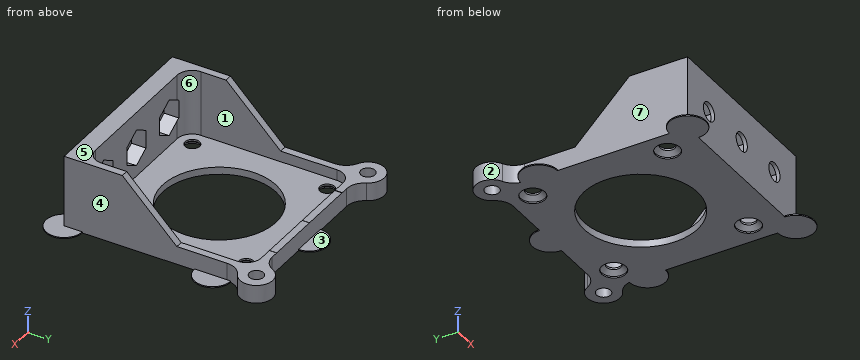
from build123d import *
from build123d.topology import SkipClean

# Parameters (mm, degrees)
SKETCH3_R                                     = 19.812
SKETCH3_R_2                                   = 2.55
BOSS_EXTRUDE1_DEPTH                           = 2.54
BOSS_EXTRUDE6_DEPTH                           = 3.81
BOSS_EXTRUDE10_DEPTH                          = 22.86
BOSS_EXTRUDE10_DEPTH_BACK                     = 2.54
CHAMFER1_SIZE                                 = 20.32
CUT_EXTRUDE2_DEPTH                            = 5.08
CUT_EXTRUDE2_DEPTH_BACK                       = 73.755970889
F_1_4_CLEARANCE_HOLE1_D                       = 6.5278
SKETCH22_R                                    = 2.413
BOSS_EXTRUDE18_DEPTH                          = 6.35
FILLET1_R                                     = 6.35
CSK_FOR_FLAT_HEAD_MACHINE_SCREW_100_1_A_COUNT = 2
CSK_FOR_FLAT_HEAD_MACHINE_SCREW_100_1_A_PITCH = 47.14
CSK_FOR_FLAT_HEAD_MACHINE_SCREW_100_2_COUNT   = 2
CSK_FOR_FLAT_HEAD_MACHINE_SCREW_100_2_PITCH   = 66.66602733
CSK_FOR_FLAT_HEAD_MACHINE_SCREW_100_3_COUNT   = 2
CSK_FOR_FLAT_HEAD_MACHINE_SCREW_100_3_PITCH   = 47.14
F_10_CLEARANCE_HOLE1_D                        = 4.9784
SKETCH6_R                                     = 6.35
TABS_DEPTH                                    = 0.4


with BuildPart() as part:
    # Sketch3 → Boss-Extrude1 (new body)
    with BuildSketch(Plane.XY):
        with BuildLine():
            Line((23.755, 31.502), (-23.755, 31.502))
            ThreePointArc((-23.755, 31.502), (-29.232956234, 29.232956234), (-31.502, 23.755))
            Line((-31.502, 23.755), (-31.502, -23.755))
            ThreePointArc((-31.502, -23.755), (-29.232956234, -29.232956234), (-23.755, -31.502))
            Line((-23.755, -31.502), (23.755, -31.502))
            ThreePointArc((23.755, -31.502), (29.232956234, -29.232956234), (31.502, -23.755))
            Line((31.502, -23.755), (31.502, 23.755))
            ThreePointArc((31.502, 23.755), (29.232956234, 29.232956234), (23.755, 31.502))
        make_face()
        Circle(SKETCH3_R, mode=Mode.SUBTRACT)
        with Locations((23.57, 23.57)):
            Circle(SKETCH3_R_2, mode=Mode.SUBTRACT)
        with Locations((-23.57, 23.57)):
            Circle(SKETCH3_R_2, mode=Mode.SUBTRACT)
        with Locations((-23.57, -23.57)):
            Circle(SKETCH3_R_2, mode=Mode.SUBTRACT)
        with Locations((23.57, -23.57)):
            Circle(SKETCH3_R_2, mode=Mode.SUBTRACT)
    extrude(amount=BOSS_EXTRUDE1_DEPTH)

    # Sketch16 → Boss-Extrude6 (add)
    with BuildSketch(Plane.XY.offset(2.54)):
        with BuildLine():
            Line((23.755, 31.502), (-23.755, 31.502))
            ThreePointArc((-23.755, 31.502), (-29.232956234, 29.232956234), (-31.502, 23.755))
            Line((-31.502, 23.755), (-31.502, -23.755))
            ThreePointArc((-31.502, -23.755), (-29.232956234, -29.232956234), (-23.755, -31.502))
            Line((-23.755, -31.502), (23.755, -31.502))
            ThreePointArc((23.755, -31.502), (29.232956234, -29.232956234), (31.502, -23.755))
            Line((31.502, -23.755), (31.502, 23.755))
            ThreePointArc((31.502, 23.755), (29.232956234, 29.232956234), (23.755, 31.502))
        make_face()
        with BuildLine():
            Line((23.755, 28.962), (-23.755, 28.962))
            ThreePointArc((-23.755, 28.962), (-27.43690501, 27.43690501), (-28.962, 23.755))
            Line((-28.962, 23.755), (-28.962, -23.755))
            ThreePointArc((-28.962, -23.755), (-27.43690501, -27.43690501), (-23.755, -28.962))
            Line((-23.755, -28.962), (23.755, -28.962))
            ThreePointArc((23.755, -28.962), (27.43690501, -27.43690501), (28.962, -23.755))
            Line((28.962, -23.755), (28.962, 23.755))
            ThreePointArc((28.962, 23.755), (27.43690501, 27.43690501), (23.755, 28.962))
        make_face(mode=Mode.SUBTRACT)
    extrude(amount=BOSS_EXTRUDE6_DEPTH)

    # Sketch17 → Boss-Extrude10 (add, two sides: drawn at the far end of the back side and taken through both)
    with SkipClean():  # the faces are left unmerged after this step: merging them gives an invalid solid
        with BuildSketch(Plane.XY.offset(2.54).offset(-BOSS_EXTRUDE10_DEPTH_BACK)):
            with BuildLine():
                Line((-31.502, -35.312), (31.502, -35.312))
                Line((31.502, -35.312), (31.502, -16.262))
                Line((31.502, -16.262), (28.962, -16.262))
                Line((28.962, -16.262), (28.962, -23.755))
                ThreePointArc((28.962, -23.755), (27.43690501, -27.43690501), (23.755, -28.962))
                Line((23.755, -28.962), (-23.755, -28.962))
                ThreePointArc((-23.755, -28.962), (-27.43690501, -27.43690501), (-28.962, -23.755))
                Line((-28.962, -23.755), (-28.962, -16.262))
                Line((-28.962, -16.262), (-31.502, -16.262))
                Line((-31.502, -16.262), (-31.502, -35.312))
            make_face()
        extrude(amount=BOSS_EXTRUDE10_DEPTH + BOSS_EXTRUDE10_DEPTH_BACK)
    add(part.part.scale(1), mode=Mode.REPLACE)  # the faces are merged on a copy

    # Chamfer1
    # the kernel refuses this chamfer: 20.32 mm, written as the material it adds along each edge
    with BuildSketch(Plane(origin=(28.962, -16.262, 6.35), x_dir=(0, -0.02749587661058643, 0.9996219169112968), z_dir=(1, 0, 0))) as chamfer1_piece_1_section:
        Polygon((CHAMFER1_SIZE * 0.999621916911, -CHAMFER1_SIZE * 0.0274958766106), (-CHAMFER1_SIZE * 0.0274958766106, -CHAMFER1_SIZE * 0.999621916911), (0, 0), align=None)
    chamfer1_piece_1 = extrude(amount=2.54, mode=Mode.PRIVATE)
    chamfer1_piece_1 = split(chamfer1_piece_1, bisect_by=Plane(origin=(30.232, -9.48984053, 25.4), z_dir=(0, 0, -1)), keep=Keep.TOP, mode=Mode.PRIVATE)
    add(chamfer1_piece_1)
    with BuildSketch(Plane(origin=(-31.502, -16.262, 6.35), x_dir=(0, -0.02749587661058643, 0.9996219169112968), z_dir=(1, 0, 0))) as chamfer1_piece_2_section:
        Polygon((CHAMFER1_SIZE * 0.999621916911, -CHAMFER1_SIZE * 0.0274958766106), (-CHAMFER1_SIZE * 0.0274958766106, -CHAMFER1_SIZE * 0.999621916911), (0, 0), align=None)
    chamfer1_piece_2 = extrude(amount=2.54, mode=Mode.PRIVATE)
    chamfer1_piece_2 = split(chamfer1_piece_2, bisect_by=Plane(origin=(-30.232, -9.48984053, 25.4), z_dir=(0, 0, -1)), keep=Keep.TOP, mode=Mode.PRIVATE)
    add(chamfer1_piece_2)

    # Sketch18 → Cut-Extrude2 (cut, two sides: drawn at the far end of the back side and taken through both)
    with BuildSketch(Plane.XZ.offset(28.962).offset(-CUT_EXTRUDE2_DEPTH_BACK)):
        Polygon((0, 19.079143124), (-5.5245, 15.889571562), (-5.5245, 9.510428438), (0, 6.320856876), (5.5245, 9.510428438), (5.5245, 15.889571562), align=None)
        Polygon((-24.5745, 15.889571562), (-19.05, 19.079143124), (-13.5255, 15.889571562), (-13.5255, 9.510428438), (-19.05, 6.320856876), (-24.5745, 9.510428438), align=None)
        Polygon((19.05, 19.079143124), (13.5255, 15.889571562), (13.5255, 9.510428438), (19.05, 6.320856876), (24.5745, 9.510428438), (24.5745, 15.889571562), align=None)
    extrude(amount=CUT_EXTRUDE2_DEPTH + CUT_EXTRUDE2_DEPTH_BACK, mode=Mode.SUBTRACT)

    # 1/4 Clearance Hole1 (through all)
    with Locations(Plane(origin=(0, -34.042, 0), x_dir=(1, 0, 0), z_dir=(0, 1, 0))):
        with Locations((-19.05, -12.7), (0, -12.7), (19.05, -12.7)):
            Hole(F_1_4_CLEARANCE_HOLE1_D / 2)

    # Sketch22 → Boss-Extrude18 (add)
    with BuildSketch(Plane(origin=(0, 0, 0), x_dir=(-1, 0, 0), z_dir=(0, 0, -1))):
        with BuildLine():
            ThreePointArc((-27.002557269, 30.78844729), (-26.814125955, 31.617757649), (-26.750848437, 32.465848437))
            ThreePointArc((-26.750848437, 32.465848437), (-37.061910478, 35.862528982), (-30.78844729, 27.002557269))
            ThreePointArc((-30.78844729, 27.002557269), (-29.232956234, 29.232956234), (-27.002557269, 30.78844729))
        make_face()
        with Locations((-32.465848437, 32.465848437)):
            Circle(SKETCH22_R, mode=Mode.SUBTRACT)
    boss_extrude18 = extrude(amount=-BOSS_EXTRUDE18_DEPTH)

    # Mirror3: Boss-Extrude18 across plane
    add(boss_extrude18.mirror(Plane(origin=(0, 0, 0), x_dir=(0, 0, 1), z_dir=(1, 0, 0))))

    # Fillet1
    fillet1_edges = [part.edges().sort_by_distance(p)[0] for p in [
        (27.002557269, 30.78844729, 3.175),
        (30.78844729, 27.002557269, 3.175),
        (-27.002557269, 30.78844729, 3.175),
        (-30.78844729, 27.002557269, 3.175),
    ]]
    fillet(fillet1_edges, radius=FILLET1_R)

    # Sketch23 → CSK for  Flat Head Machine Screw (100)1 (revolve, cut)
    with BuildSketch(Plane(origin=(23.57, 23.57, 0), x_dir=(0, 1, 0), z_dir=(1, 0, 0))):
        Polygon((0, 0), (0, 25.4), (2.4892, 25.4), (2.4892, 1.957292137), (4.216399111, 0.508), (4.216399111, 0), align=None)
    csk_for_flat_head_machine_screw_100_1 = revolve(axis=Axis((23.57, 23.57, -6.35), (0, 0, 1)), mode=Mode.SUBTRACT)

    # CSK for  Flat Head Machine Screw (100)1 a: CSK for  Flat Head Machine Screw (100)1 ×2
    with Locations(*[(-i * CSK_FOR_FLAT_HEAD_MACHINE_SCREW_100_1_A_PITCH, 0, 0) for i in range(1, CSK_FOR_FLAT_HEAD_MACHINE_SCREW_100_1_A_COUNT)]):
        add(csk_for_flat_head_machine_screw_100_1, mode=Mode.SUBTRACT)

    # CSK for Flat Head Machine Screw _100 2: CSK for  Flat Head Machine Screw (100)1 ×2
    with Locations(*[Vector(-0.7071067811865476, -0.7071067811865476, 0) * (i * CSK_FOR_FLAT_HEAD_MACHINE_SCREW_100_2_PITCH) for i in range(1, CSK_FOR_FLAT_HEAD_MACHINE_SCREW_100_2_COUNT)]):
        add(csk_for_flat_head_machine_screw_100_1, mode=Mode.SUBTRACT)

    # CSK for Flat Head Machine Screw _100 3: CSK for  Flat Head Machine Screw (100)1 ×2
    with Locations(*[(0, -i * CSK_FOR_FLAT_HEAD_MACHINE_SCREW_100_3_PITCH, 0) for i in range(1, CSK_FOR_FLAT_HEAD_MACHINE_SCREW_100_3_COUNT)]):
        add(csk_for_flat_head_machine_screw_100_1, mode=Mode.SUBTRACT)

    # #10 Clearance Hole1 (through all)
    with Locations(Plane(origin=(0, 0, 0), x_dir=(-1, 0, 0), z_dir=(0, 0, -1))):
        with Locations((-32.465848437, 32.465848437), (32.465848437, 32.465848437)):
            Hole(F_10_CLEARANCE_HOLE1_D / 2)

    # Sketch6 → Tabs (add)
    with BuildSketch(Plane(origin=(0, -30.232, 0), x_dir=(-1, 0, 0), z_dir=(0, 0, -1))):
        with Locations((31.502, -5.08)):
            Circle(SKETCH6_R)
        with Locations((-31.502, -5.08)):
            Circle(SKETCH6_R)
        with Locations((-31.502, 46.821157202)):
            Circle(SKETCH6_R)
        with Locations((31.502, 46.821157202)):
            Circle(SKETCH6_R)
        with Locations((0, 61.734)):
            Circle(SKETCH6_R)
    extrude(amount=-TABS_DEPTH)


solid = part.part
Work out the finished part from the listing and answer in its coordinate system (mm). Face numbers are marked on the shaded views. A direction names the side the tool comes from. Give positions to 0.01 mm unless a question says otherwise; leave off trailing zeros. Write each loop counter-clockwise with the first axis right and the second up, starting at its lowest first coordinate (ties: lowest second). Pieces come first, ordered by that corner, then holes. Notation, with made-up numbers: (34, -19) - (61, -19) arc R20 ccw to (61, -7) - close; hole circle Ø2 at (34, -0.5). An arc over 180 degrees is marked (long way). One line per item, written item: value. Start each with the question number.
1. Find section B-B (z = 12.7). State how many separate pieces and enclosed holes the cut face has, then the cut area to 3 significant figures.
2. Find section C-C (z = 22.25). Write down the section's boundary in (x, y) (3 decimals), then the cut area to 3 significant figures.
3. Consider probe 1 along X at (y, z) = (-16.5, 22.75); probe 2 along Y at (x, z) = (23.57, 2.45); probe 3 along Z at (x, y) = (-19, -34). Determine where each line is inside the solid, lowest interval first.
4. Find section A-A (y = 0). Write down the section's boundary in (x, z), then the cut area to 3 significant figures.
5. Given pin 1 (3 mm diameter, centred on x = -23.57, y = -23.57, fed in from -Z); pin 2 (4 mm diameter, centred on x = 5, y = 24, fed in from +Z); pin 3 (5.5 mm diameter, centred on x = 20, z = 16, fed in from +Y); pin 4 (12 mm diameter, centred on y = -25.5, z = 19.5, fed in from -X), each flat-ended and moving along its own axis, determine where each tip first touches the part or whether it passes through.
6. Find section D-D (y = 18). Write down the section's boundary in (x, z), then the cut area to 3 significant figures.
7. For the marked faces 1, 2 and 3, determine the directions among +Z, -Z, +X, -X, +Y, -Y from which every point of the face is accessible in a straight line to the end or side of a thin tool.
8. For a pull along X with two mould halves and no side action, classify the marked faces 4, 5, 6 and 7 as +X half, -X half, draft (parallel to the pull), parting line (faces both ways), or undercut.
Geometry results:
1. separate pieces: 4
1. enclosed holes: 0
1. area: 354 mm2
2. outline: (-31.502, -35.312) - (31.502, -35.312) - (31.502, -11.842) - (28.962, -11.842) - (28.962, -23.755) arc R5.207 cw to (23.755, -28.962) - (-23.755, -28.962) arc R5.207 cw to (-28.962, -23.755) - (-28.962, -11.842) - (-31.502, -11.842) - close
2. area: 499 mm2
3. probe 1: -31.5 to -28.96, 28.96 to 31.5
3. probe 2: -35.31 to -26.12, -21.02 to 21.02, 26.12 to 31.79
3. probe 3: 0 to 6.35, 19.05 to 25.4
4. outline: (-31.5, 0) - (-19.81, 0) - (-19.81, 2.54) - (-28.96, 2.54) - (-28.96, 10.41) - (-31.5, 10.41) - close; (19.81, 0) - (31.5, 0) - (31.5, 10.41) - (28.96, 10.41) - (28.96, 2.54) - (19.81, 2.54) - close
4. area: 99.4 mm2
5. pin 1: through
5. pin 2: z = 2.54
5. pin 3: y = -28.96
5. pin 4: x = -31.5
6. outline: (-37.69, 0) - (-8.28, 0) - (-8.28, 2.54) - (-28.96, 2.54) - (-28.96, 6.35) - (-31.5, 6.35) - (-31.5, 0.4) - (-37.69, 0.4) - close; (8.28, 0) - (37.69, 0) - (37.69, 0.4) - (31.5, 0.4) - (31.5, 6.35) - (28.96, 6.35) - (28.96, 2.54) - (8.28, 2.54) - close
6. area: 142 mm2
7. face 1: +Z
7. face 2: +Z, -Z
7. face 3: +Z, +Y
8. face 4: +X half
8. face 5: draft
8. face 6: undercut
8. face 7: -X half
